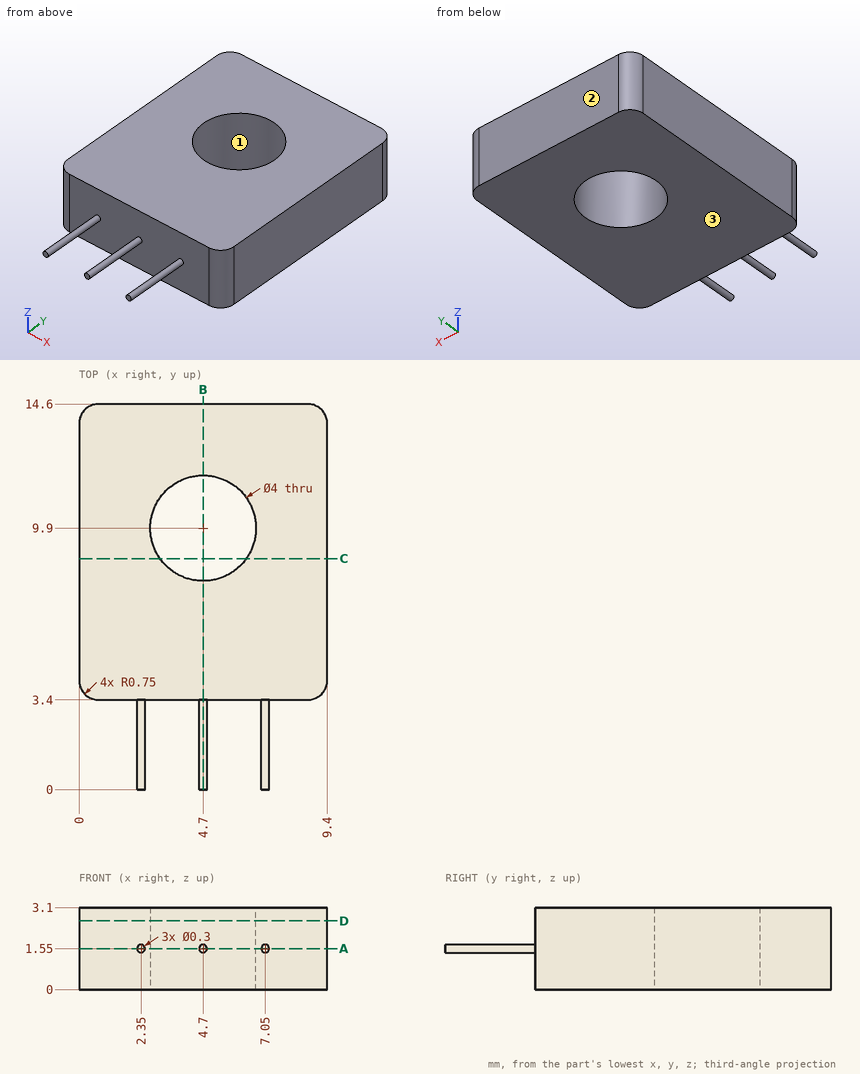
Job drawing, mm, ordinate dimensions from the low corner. One solid piece. Give positions to 0.01 mm unless a question says otherwise; leave off trailing zeros. Loops run counter-clockwise (first coordinate to the right, second up) from the corner with the lowest first, then second, coordinate; pieces in that order, holes last. Notation, with made-up numbers: (53, 11) -> (81, 11) arc R15 cw to (81, 29) -> close; hole circle Ø5 at (-19, 37.25). An arc over 180 degrees is marked (long way). Use a Markdown table: item, result. Add a question column.
(1) Mould opens along Y. For the marked faces 1, 2 and 3 say: +Y half, -Y half, draft (parallel to the pull), parting line (faces both ways), or undercut.
(2) Slice it at D-D on z = 2.6. List the corners of the cut face in (x, y), and give its area (3 significant figures).
(3) Slice it at C-C on y = 8.75. List the corners of the cut face in (x, z), and give its area (3 significant figures).
(4) Slice it at A-A on z = 1.55. List the corners of the cut face in (x, y), and give its area (3 significant figures).
(5) Wall check: line 1 along Y through (x, z) = (4.7, 2.25); line 2 along X through (y, z) = (9.9, 0.65); line 3 along Y through (x, z) = (7.5, 0.5). Give the ranges that are in metal, low to high.
(6) Drop flat-ended pins along their axis: pin 1 Ø3.5 at (x, y) = (4.7, 9.9) entering from -Z; pin 2 Ø0.9 at (x, z) = (6, 1.5) entering from -Y. Give the stop position or say it passes through.
(7) Slice it at B-B on x = 4.7. List the corners of the cut face in (y, z).
Filled sheet:
| question | item | result |
|---|---|---|
| 1 | face 1 | undercut |
| 1 | face 2 | +Y half |
| 1 | face 3 | draft |
| 2 | outline | (0, 4.15) arc R0.75 ccw to (0.75, 3.4) -> (8.65, 3.4) arc R0.75 ccw to (9.4, 4.15) -> (9.4, 13.85) arc R0.75 ccw to (8.65, 14.6) -> (0.75, 14.6) arc R0.75 ccw to (0, 13.85) -> close; hole circle Ø4 at (4.7, 9.9) |
| 2 | area | 92.2 mm2 |
| 3 | outline | (0, 0) -> (3.06, 0) -> (3.06, 3.1) -> (0, 3.1) -> close; (6.34, 0) -> (9.4, 0) -> (9.4, 3.1) -> (6.34, 3.1) -> close |
| 3 | area | 19.0 mm2 |
| 4 | outline | (0, 4.15) arc R0.75 ccw to (0.75, 3.4) -> (2.2, 3.4) -> (2.2, 0) -> (2.5, 0) -> (2.5, 3.4) -> (4.55, 3.4) -> (4.55, 0) -> (4.85, 0) -> (4.85, 3.4) -> (6.9, 3.4) -> (6.9, 0) -> (7.2, 0) -> (7.2, 3.4) -> (8.65, 3.4) arc R0.75 ccw to (9.4, 4.15) -> (9.4, 13.85) arc R0.75 ccw to (8.65, 14.6) -> (0.75, 14.6) arc R0.75 ccw to (0, 13.85) -> close; hole circle Ø4 at (4.7, 9.9) |
| 4 | area | 95.3 mm2 |
| 5 | line 1 | 3.4 to 7.9, 11.9 to 14.6 |
| 5 | line 2 | 0 to 2.7, 6.7 to 9.4 |
| 5 | line 3 | 3.4 to 14.6 |
| 6 | pin 1 | through |
| 6 | pin 2 | y = 3.4 |
| 7 | outline | (0, 1.4) -> (3.4, 1.4) -> (3.4, 0) -> (7.9, 0) -> (7.9, 3.1) -> (3.4, 3.1) -> (3.4, 1.7) -> (0, 1.7) -> close; (11.9, 0) -> (14.6, 0) -> (14.6, 3.1) -> (11.9, 3.1) -> close |
